Work out the finished part from the listing and answer in its coordinate system (mm). Coordinates: 2 decimals unless noted, no trailing zeros. Order: outer loops, then holes, each group sorted by start corner. A loop starts at its lowest first (then second) coordinate and runs counter-clockwise, first axis right, second up. Notation, with made-up numbers: (67.5, 28.25) -> (90.5, 28.25) arc R15 cw to (90.5, 34.25) -> close; hole circle Ø2 at (51, 14). An arc over 180 degrees is marked (long way). Write item = value, one per line. Start each with the question number.
Q1. The part is cut by section A-A, the plane y = 0.8. Determine the outline of the cut face in (x, z).
Q2. The part is cut by section B-B, the plane x = -40. Determine the outline of the cut face in (y, z), plus the area to 3 significant figures.
Q3. Straight lines are drawn through the part: L1, parallel to Z at x = -40, y = 0.3; L2, parallel to X at y = 0.85, z = -20; L3, parallel to X at y = 0.3, z = -15. For each, find the intervals that lie inside material, in ascending order. Write a range as from..to.
Q4. The part is cut by section D-D, the plane z = -13. Determine the outline of the cut face in (x, y), plus the area to 3 significant figures.
Q5. The part is cut by section C-C, the plane z = -20. Determine the outline of the cut face in (x, y).
Q6. For a pull along Z with two mould halves and no side action, classify faces 1 (the flat face through (-37, 0, -20)), 2 (the cylindrical face through (-12.998, 0.507, -20.306)) as +Z half, -Z half, draft (parallel to the pull), parting line (faces both ways), or undercut.
Autodesk Inventor part; units mm, degrees
ref_plane "YZ Plane" through (0, 0, 0) normal (1, 0, 0) x (0, 1, 0)
ref_plane "XZ Plane" through (0, 0, 0) normal (0, 1, 0) x (-1, 0, 0)
ref_plane "XY Plane" through (0, 0, 0) normal (0, 0, 1) x (1, 0, 0)
sketch "Boceto1" plane through (0, 0, 0) normal (0, 1, 0) x (-1, 0, 0)
  line L0 (0, 0) -> (0, -40)
  line L1 (0, -40) -> (60, -40)
  line L2 (60, 0) -> (0, 0)
  line L3 (60, -40) -> (60, 0)
  dimension "d1" = 60
  dimension "d3" = 40
extrude "Extrusión1" add sketch "Boceto1" along normal blind 1
sketch "Boceto2" plane through (0, 0, 0) normal (0, -1, 0) x (1, 0, 0)
  line L0 (0, 0) -> (0, -40)
  circle A0 centre (9, -20) radius 22
  point P0 (0, -20)
  dimension "d7" = 44
  dimension "d8" = 9
extrude "Extrusión2" cut sketch "Boceto2" against normal through all
sketch "Boceto3" plane through (0, 1, 0) normal (0, 1, 0) x (1, 0, 0)
  arc A0 (-0.1652, 40) -> (-0.1652, 0) centre (9, 20) ccw
  line L0 (-0.1652, 40) -> (-60, 40)
  line L1 (-60, 40) -> (-60, 0)
  line L2 (-60, 0) -> (-0.1652, 0)
  line L3 (-60, 40) -> (-3, 40)
  line L4 (-3, 40) -> (-3, 0)
  line L5 (-3, 0) -> (-60, 0)
  line L6 (-60, 0) -> (-60, 40)
  point P0 (0, 0)
  point P1 (-3, 38.4391)
  point P2 (-3, 1.5609)
  dimension "d11" = 57
extrude "Extrusión3" cut sketch "Boceto3" against normal through all contours A0 L4 L2 L1 L0 keep common part
sketch "Boceto4" plane through (0, 0, 0) normal (0, -1, 0) x (1, 0, 0)
  point P0 (-40, -20)
hole "Agujero1" at (-40, 0, -20) direction (0, 1, 0) diameter 3.4 end through all
properties part number "platina_1"
Model answer:
q1.outline = (-60, -40) -> (-3, -40) -> (-3, -38.44) arc R22 cw to (-3, -1.56) -> (-3, 0) -> (-60, 0) -> close; hole circle Ø3.4 at (-40, -20)
q2.outline = (0, -40) -> (1, -40) -> (1, -21.7) -> (0, -21.7) -> close; (0, -18.3) -> (1, -18.3) -> (1, 0) -> (0, 0) -> close
q2.area = 36.6 mm2
q3.L1 = -40..-21.7, -18.3..0
q3.L2 = -60..-41.7, -38.3..-13
q3.L3 = -60..-12.42
q4.outline = (-60, 0) -> (-11.86, 0) -> (-11.86, 1) -> (-60, 1) -> close
q4.area = 48.1 mm2
q5.outline = (-60, 0) -> (-41.7, 0) -> (-41.7, 1) -> (-60, 1) -> close; (-38.3, 0) -> (-13, 0) -> (-13, 1) -> (-38.3, 1) -> close
q6.face_1 = draft
q6.face_2 = undercut
